For this review, take the finished solid that the model builds, in its own axes (mm). Face numbers are marked on the shaded views. A direction names the side the tool comes from. Give positions to 0.01 mm unless a question says otherwise; leave off trailing zeros. Write each loop counter-clockwise with the first axis right and the second up, starting at its lowest first coordinate (ties: lowest second). Pieces come first, ordered by that corner, then holes. Notation, with made-up numbers: (-9.5, -19) -> (15.5, -19) arc R31 cw to (15.5, 15) -> close; hole circle Ø4 at (-16, 65.25). An arc over 180 degrees is marked (long way). Return JSON: item names as keys, results as strings.
from build123d import *

# Parameters (mm, degrees)
BOSS_EXTRUDE1_DEPTH     = 8
SKETCH2_R               = 1.25
BOSS_EXTRUDE2_DEPTH     = 4
M2_5_TAPPED_HOLE1_D     = 2.05
M2_5_TAPPED_HOLE1_DEPTH = 5.5
M2_5_TAPPED_HOLE1_TIP   = 0.615882135


with BuildPart() as part:
    # Sketch1 → Boss-Extrude1 (new body)
    with BuildSketch(Plane.XY):
        Polygon((-1.154700538, -2), (1.154700538, -2), (2.309401077, 0), (1.154700538, 2), (-1.154700538, 2), (-2.309401077, 0), align=None)
    extrude(amount=BOSS_EXTRUDE1_DEPTH)

    # Sketch2 → Boss-Extrude2 (add)
    with BuildSketch(Plane.XY.offset(8)):
        Circle(SKETCH2_R)
    extrude(amount=BOSS_EXTRUDE2_DEPTH)

    # M2.5 Tapped Hole1
    with Locations(Plane(origin=(0, 0, 0), x_dir=(-1, 0, 0), z_dir=(0, 0, -1))):
        with Locations((0, 0)):
            Hole(M2_5_TAPPED_HOLE1_D / 2, depth=M2_5_TAPPED_HOLE1_DEPTH)
            with Locations((0, 0, -(M2_5_TAPPED_HOLE1_DEPTH + M2_5_TAPPED_HOLE1_TIP / 2))):  # 118° drill point
                Cone(0, M2_5_TAPPED_HOLE1_D / 2, M2_5_TAPPED_HOLE1_TIP, mode=Mode.SUBTRACT)


solid = part.part
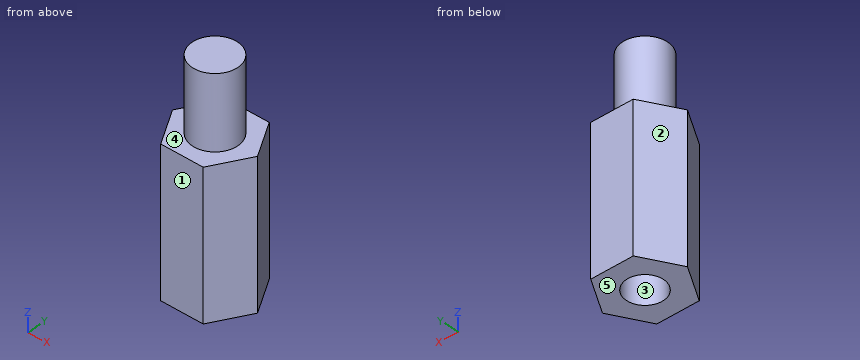
1. Add section B-B, the plane z = 8.5. State the section outline as (x, y) points.
Results found:
{"outline": "circle Ø2.5 at (0, 0)"}
2. Add section A-A, the plane z = 3. State the section outline as (x, y) points (3 decimals), plus the area to 3 significant figures.
Results found:
{"outline": "(-2.309, 0) -> (-1.155, -2) -> (1.155, -2) -> (2.309, 0) -> (1.155, 2) -> (-1.155, 2) -> close; hole circle Ø2.05 at (0, 0)", "area": "10.6 mm²"}
3. Add section D-D, the plane y = -1.65. State the section outline as (x, z) points.
Results found:
{"outline": "(-1.36, 0) -> (1.36, 0) -> (1.36, 8) -> (-1.36, 8) -> close"}
4. The part is to be moulded in two halves that separate along Y. For the marked faces 1, 2 and 3, say which applies: +Y half, -Y half, draft (parallel to the pull), parting line (faces both ways), or undercut.
Results found:
{"face 1": "-Y half", "face 2": "+Y half", "face 3": "undercut"}
5. For the marked faces 4 and 5, list the 3-axis set-ups (+Z, -Z, +X, -X, +Y, -Y) from which the entire face can be reached by the end or side of a thin tool; tool diameter is ignored.
Results found:
{"face 4": "+Z", "face 5": "-Z, +X, -X, +Y, -Y"}
6. To check wall thickness, follow probe 1 along Y at (x, z) = (0, 3.45) (3 decimals); probe 2 along X at (y, z) = (-0.05, 5); probe 3 along Z at (x, y) = (1.3, 0.7). State the ranges of each line that lie inside material, in increasing order.
Results found:
{"probe 1": "y = -2 to -1.025, 1.025 to 2", "probe 2": "x = -2.28 to -1.02, 1.02 to 2.28", "probe 3": "z = 0 to 8"}
7. Add section C-C, the plane x = 1.8. State the section outline as (y, z) points, plus the area to 3 significant figures.
Results found:
{"outline": "(-0.88, 0) -> (0.88, 0) -> (0.88, 8) -> (-0.88, 8) -> close", "area": "14.1 mm²"}
8. For pin 1 (1 mm diameter, centred on x = 1, y = -1, fed in from -Z), flat-tipped, find the tip position at first contact; note if it passes through.
Results found:
{"pin 1": "stops at z = 0"}
